Verification items for this drawing (mm, ordinates from the low corner). Coordinates: 2 decimals unless noted, no trailing zeros. Order: outer loops, then holes, each group sorted by start corner. A loop starts at its lowest first (then second) coordinate and runs counter-clockwise, first axis right, second up.
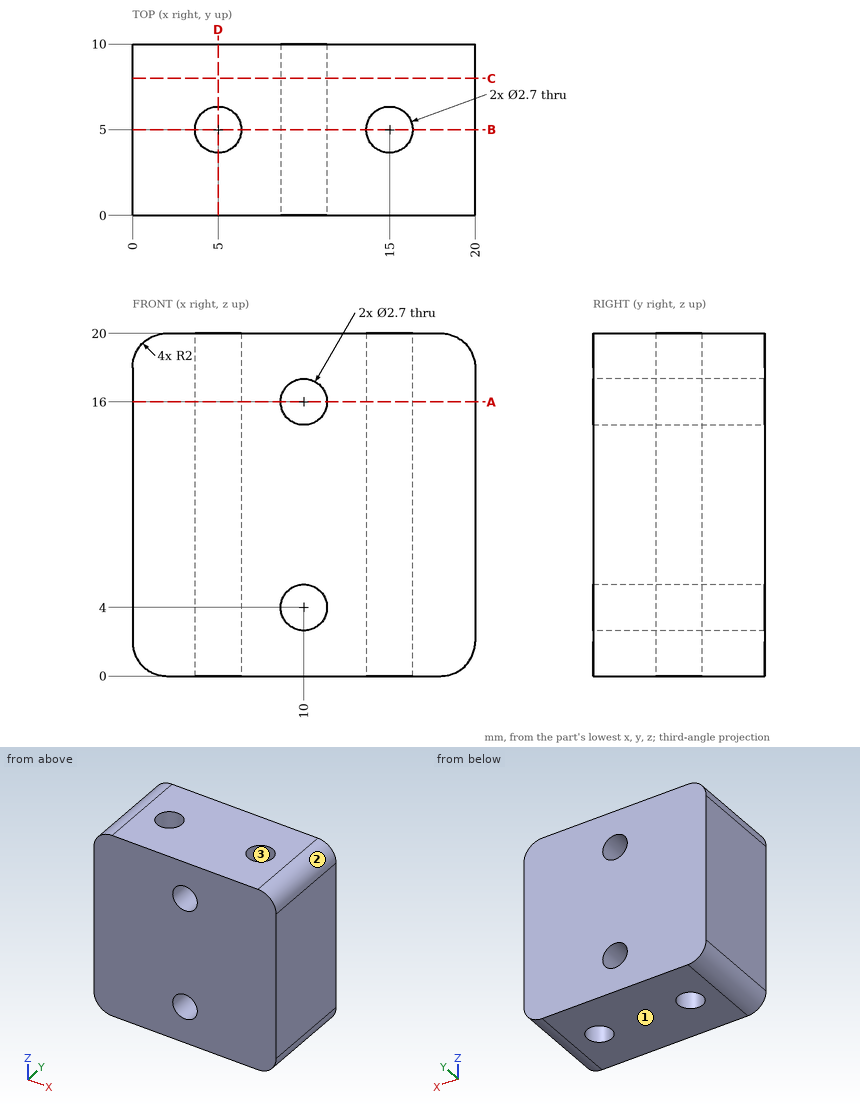
Item 1: Sectioned sample at C-C (y = 8). Record the cut outline in (x, z).
Item 2: Depth check by flat-ended pin: P1, Ø1.6, axis at x = 15, y = 5, coming from the -Z side. Enter the tip coordinate at first touch or a pass-through.
Item 3: Sectioned sample at D-D (x = 5). Record the cut outline in (y, z), and give its area (3 significant figures).
Item 4: Sectioned sample at B-B (y = 5). Record the cut outline in (x, z).
Item 5: Thickness scan on line 1 along X through (y, z) = (7.25, 16); line 2 along X through (y, z) = (5.75, 4); line 3 along Y through (x, z) = (15, 4). Record the ranges inside material, lowest first.
Item 6: Release check for a two-part mould opening along X. For the marked faces 1, 2 and 3 record: pulls with the +X half, pulls with the -X half, needs draft (parallel to the pull), parting line crosses it, or undercut.
Item 7: Sectioned sample at A-A (z = 16). Record the cut outline in (x, y), and give its area (3 significant figures).
Geometry check:
1. outline: (0, 2) arc R2 ccw to (2, 0) - (18, 0) arc R2 ccw to (20, 2) - (20, 18) arc R2 ccw to (18, 20) - (2, 20) arc R2 ccw to (0, 18) - close; hole circle Ø2.7 at (10, 4); hole circle Ø2.7 at (10, 16)
2. P1: passes through
3. outline: (0, 0) - (3.65, 0) - (3.65, 20) - (0, 20) - close; (6.35, 0) - (10, 0) - (10, 20) - (6.35, 20) - close
3. area: 146 mm2
4. outline: (0, 2) arc R2 ccw to (2, 0) - (3.65, 0) - (3.65, 20) - (2, 20) arc R2 ccw to (0, 18) - close; (6.35, 0) - (13.65, 0) - (13.65, 20) - (6.35, 20) - close; (16.35, 0) - (18, 0) arc R2 ccw to (20, 2) - (20, 18) arc R2 ccw to (18, 20) - (16.35, 20) - close; hole circle Ø2.7 at (10, 4); hole circle Ø2.7 at (10, 16)
5. line 1: x = 0 to 8.65, 11.35 to 20
5. line 2: x = 0 to 3.88, 6.12 to 8.65, 11.35 to 13.88, 16.12 to 20
5. line 3: y = 0 to 3.65, 6.35 to 10
6. face 1: needs draft
6. face 2: pulls with the +X half
6. face 3: undercut
7. outline: (0, 0) - (8.65, 0) - (8.65, 10) - (0, 10) - close; (11.35, 0) - (20, 0) - (20, 10) - (11.35, 10) - close; hole circle Ø2.7 at (5, 5); hole circle Ø2.7 at (15, 5)
7. area: 162 mm2
